Autodesk Fusion 360 part; units mm, degrees
sketch "Sketch1" plane through (0, 0, 0) normal (0, 0, 1) x (1, 0, 0)
  circle A0 centre (0, 0) radius 5.125
  circle A1 centre (0, 0) radius 6
  circle A2 centre (0, 0) radius 7.5
  dimension "d1" = 10.25
  dimension "d2" = 12
  dimension "d3" = 15
extrude "Extrude1" add sketch "Sketch1" along normal blind 3 contours A2
extrude "Extrude2" add sketch "Sketch1" along normal blind 9 contours A1
chamfer "Chamfer1" distance 1 angle 45 1 edges at (-6.9925, -2.7121, 0)
thread "Thread1" thread offset 0 thread length 10
CAD build for the part. Positions are in the model's coordinates, mm. A direction names the side the tool comes from. Coordinates: 2 decimals unless noted, no trailing zeros. Write each loop counter-clockwise with the first axis right and the second up, starting at its lowest first coordinate (ties: lowest second). Pieces come first, ordered by that corner, then holes. Notation, with made-up numbers: M 67,-29 L 119,-29 A22 ccw 119,8 Z; hole C 1,86.5 d10. An arc over 180 degrees is marked long. Answer as a JSON object with one key per item and string values. Group by question number.
1) Mould opens along X. For faces 3 (the face through (-1.111, 5.003, 4.437)), 4 (the face through (-7.493, -0.33, 1.986)), 5 (the face through (5, 2, 9)) say: +X half, -X half, draft (parallel to the pull), parting line (faces both ways), or undercut.
2) Saw through at A-A (x = 0). Write the cut outline in (y, z) (3 decimals), plus the area to 4 significant figures.
3) Saw through at D-D (z = 3.5). Write the cut outline in (x, y) (3 decimals).
4) Saw through at C-C (z = 2). Write the cut outline in (x, y) (3 decimals).
5) Wall check: line 1 (Y direction, x = 0, z = 3.5) (3 decimals); line 2 (Y direction, x = 0, z = 2) (3 decimals); line 3 (X direction, y = 1.5, z = 3.75). Give the ranges that are in metal, low to high. Write a range as from..to.
6) Tool access for faces 1 (the face through (-6, 0, 6)), 2 (the face through (5, 2, 0)): list every direction of +Z, -Z, +X, -X, +Y, -Y with a clear straight run to the whole face (end or side of a thin tool).
7) Pin check, flat tips, straight feed: pin 1 Ø5 at (x, y) = (0.5, 1.5) entering from +Z; pin 2 Ø4 at (y, z) = (1, 5.5) entering from -X; pin 3 Ø4 at (x, y) = (4, 1.5) entering from -Z; pin 4 Ø5 at (y, z) = (-5.5, 7.5) entering from -X. Stop position of each tip, or through.
Values follow:
{
 "1": {"face 3": "undercut", "face 4": "parting line", "face 5": "draft"},
 "2": {"outline": "M -7.5,1 L -6.5,0 L -5.125,0 L -5.125,9 L -6,9 L -6,3 L -7.5,3 Z; M 5.125,0 L 6.5,0 L 7.5,1 L 7.5,3 L 6,3 L 6,9 L 5.125,9 Z", "area": "23.75 mm2"},
 "3": {"outline": "C 0,0 d12; hole C 0,0 d10.25"},
 "4": {"outline": "C 0,0 d15; hole C 0,0 d10.25"},
 "5": {"line 1": "y = -6..-5.125, 5.125..6", "line 2": "y = -7.5..-5.125, 5.125..7.5", "line 3": "x = -5.81..-4.9, 4.9..5.81"},
 "6": {"face 1": "+Z", "face 2": "-Z, +X, -X, +Y, -Y"},
 "7": {"pin 1": "passes through", "pin 2": "stops at x = -6", "pin 3": "stops at z = 0", "pin 4": "stops at x = -5.2"}
}
